from build123d import *

# Parameters (mm, degrees)
F1_DEPTH    = 15
F2_R        = 3.175
F3_DEPTH    = 25.4
F4_R        = 3.175
F5_DEPTH    = 3.96875
F6_T1_DEPTH = 3
F7_R        = 7.62


# Not quite as in the source:
# - a fillet or chamfer that OpenCascade refuses, or shapes differently, is made with other operations: its cross-section is extruded or revolved along the edge and cut away or added


with BuildPart() as f1:
    # F0 (on Top) → F1 (new body)
    with BuildSketch(Plane.XY):
        Polygon((-23.4638472274, 38), (-23.4638472274, -7), (-17.9638472274, -7), (-17.9638472274, 0), (-14.9638472274, 0), (-14.9638472274, -7), (-12.9638472274, -7), (-12.9638472274, 38), (-14.9638472274, 38), (-14.9638472274, 31), (-17.9638472274, 31), (-17.9638472274, 38), align=None)
    extrude(amount=F1_DEPTH)

    # F2 (on face) → F3 (cut)
    with BuildSketch(Plane(origin=(-23.4638472274, 0, 0), x_dir=(0, -1, 0), z_dir=(-1, 0, 0))):
        with Locations((-15.5, 7.5)):
            Circle(F2_R)
    extrude(amount=-F3_DEPTH, mode=Mode.SUBTRACT)

    # F4 (on face) → F5 (cut)
    with BuildSketch(Plane.YZ.offset(-12.9638472274)):
        Polygon((21.9154598913, 7.5665316996), (18.6501118036, 13.0892170926), (12.2346519124, 13.022685393), (9.0845401087, 7.4334683004), (12.3498881964, 1.9107829074), (18.7653480876, 1.977314607), align=None)
        with Locations((15.5, 7.5)):
            Circle(F4_R, mode=Mode.SUBTRACT)
    extrude(amount=-F5_DEPTH, mode=Mode.SUBTRACT)

    # F6: fillet of radius 7.62 on 4 edges, made by hand

    # F6_s2 → F6_t1 (cut)
    with BuildSketch(Plane.YZ.offset(-17.9638472274)):
        with BuildLine():
            ThreePointArc((7.62, 15), (2.2318463274, 12.7681536726), (0, 7.38))
            Line((0, 7.38), (-0.1524, 7.38))
            Line((-0.1524, 7.38), (-0.1524, 15.1524))
            Line((-0.1524, 15.1524), (7.62, 15.1524))
            Line((7.62, 15.1524), (7.62, 15))
        make_face()
        with BuildLine():
            ThreePointArc((23.38, 15), (28.7681536726, 12.7681536726), (31, 7.38))
            Line((31, 7.38), (31.1524, 7.38))
            Line((31.1524, 7.38), (31.1524, 15.1524))
            Line((31.1524, 15.1524), (23.38, 15.1524))
            Line((23.38, 15.1524), (23.38, 15))
        make_face()
        with BuildLine():
            ThreePointArc((0, 7.62), (2.2318463274, 2.2318463274), (7.62, 0))
            Line((7.62, 0), (7.62, -0.1524))
            Line((7.62, -0.1524), (-0.1524, -0.1524))
            Line((-0.1524, -0.1524), (-0.1524, 7.62))
            Line((-0.1524, 7.62), (0, 7.62))
        make_face()
        with BuildLine():
            ThreePointArc((31, 7.62), (28.7681536726, 2.2318463274), (23.38, 0))
            Line((23.38, 0), (23.38, -0.1524))
            Line((23.38, -0.1524), (31.1524, -0.1524))
            Line((31.1524, -0.1524), (31.1524, 7.62))
            Line((31.1524, 7.62), (31, 7.62))
        make_face()
    extrude(amount=F6_T1_DEPTH, mode=Mode.SUBTRACT)

    # F7
    f7_edges = [f1.edges().sort_by_distance(p)[0] for p in [
        (-13.963847, 38, 15),
        (-13.963847, -7, 0),
        (-20.713847, -7, 0),
        (-20.713847, 38, 15),
    ]]
    fillet(f7_edges, radius=F7_R)


solid = f1.part
For this review, take the finished solid that the model builds, in its own axes (mm). A direction names the side the tool comes from. Give positions to 0.01 mm unless a question says otherwise; leave off trailing zeros. Loops run counter-clockwise (first coordinate to the right, second up) from the corner with the lowest first, then second, coordinate; pieces in that order, holes last. Notation, with made-up numbers: (7, -23) -> (56, -23) arc R37 cw to (56, 14) -> close; hole circle Ø2 at (-13, 9). An arc over 180 degrees is marked (long way). One line per question, with ' | ' between items.
1) The part is to be moulded in two halves that separate along Z. For faces 1 (the flat face through (-17.964, -3, 8)), 2 (the flat face through (-14.9, 10.7, 10.3)), 3 (the cylindrical face through (-13.978, 35.827, 12.709)), 4 (the flat face through (-18, 20, 0)), say which applies: +Z half, -Z half, draft (parallel to the pull), parting line (faces both ways), or undercut.
Resolved:
face 1: draft | face 2: undercut | face 3: +Z half | face 4: -Z half
2) We need section D-D (x = -20.75). Write out the cut boundary in (y, z) (3 decimals).
Resolved:
outline: (-7, 7.62) arc R7.62 ccw to (0.62, 0) -> (38, 0) -> (38, 7.38) arc R7.62 ccw to (30.38, 15) -> (-7, 15) -> close; hole circle Ø6.35 at (15.5, 7.5)
3) Insertion check: pin 1 Ø2 at (x, y) = (-16.5, 6) entering from +Z. The pin has a flat end and moves straight along its axis. Give the tip position at first contact, or say it passes through.
Resolved:
pin 1: stops at z = 14.97
4) We need section A-A (x = -16.5). Write out the cut boundary in (y, z), plus the area to 3 significant figures.
Resolved:
outline: (0, 7.5) arc R7.62 ccw to (7.62, 0) -> (23.38, 0) arc R7.62 ccw to (31, 7.5) arc R7.62 ccw to (23.38, 15) -> (7.62, 15) arc R7.62 ccw to start; hole (9.08, 7.43) -> (12.35, 1.91) -> (18.77, 1.98) -> (21.92, 7.57) -> (18.65, 13.09) -> (12.23, 13.02) -> close | area: 308 mm2
5) We need section B-B (y = 15.5). Write out the cut boundary in (x, z) (3 decimals), plus the area to 3 significant figures.
Resolved:
outline: (-23.464, 0) -> (-12.964, 0) -> (-12.964, 1.943) -> (-16.933, 1.943) -> (-16.933, 4.325) -> (-23.464, 4.325) -> close; (-23.464, 10.675) -> (-16.933, 10.675) -> (-16.933, 13.057) -> (-12.964, 13.057) -> (-12.964, 15) -> (-23.464, 15) -> close | area: 71.9 mm2
6) For faces 5 (the cylindrical face through (-16.485, 28.666, 12.868)), 6 (the flat face through (-14.9, 10.7, 4.7)), 7 (the cylindrical face through (-16.485, 2.216, 2.248)), list the 3-axis set-ups (+Z, -Z, +X, -X, +Y, -Y) from which the entire face can be reached by the end or side of a thin tool; tool diameter is ignored.
Resolved:
face 5: +Z, +Y | face 6: +X | face 7: -Z, -Y
7) To check wall thickness, follow probe 1 along Z at (x, y) = (-20.75, 15.5) (3 decimals); probe 2 along X at (y, z) = (-0.5, 12); probe 3 along Y at (x, z) = (-22, 7.5) (3 decimals). State the ranges of each line that lie inside material, in increasing order.
Resolved:
probe 1: z = 0 to 4.325, 10.675 to 15 | probe 2: x = -23.46 to -17.96, -14.96 to -12.96 | probe 3: y = -6.999 to 12.325, 18.675 to 37.999
8) We need section C-C (z = 6.25). Write out the cut boundary in (x, y), plus the area to 3 significant figures.
Resolved:
outline: (-23.46, -6.88) -> (-17.96, -6.88) -> (-17.96, 0.12) -> (-14.96, 0.12) -> (-14.96, -6.88) -> (-12.96, -6.88) -> (-12.96, 9.78) -> (-16.93, 9.78) -> (-16.93, 12.58) -> (-23.46, 12.58) -> close; (-23.46, 18.42) -> (-16.93, 18.42) -> (-16.93, 21.17) -> (-12.96, 21.17) -> (-12.96, 38) -> (-14.96, 38) -> (-14.96, 30.88) -> (-17.96, 30.88) -> (-17.96, 38) -> (-23.46, 38) -> close | area: 345 mm2
